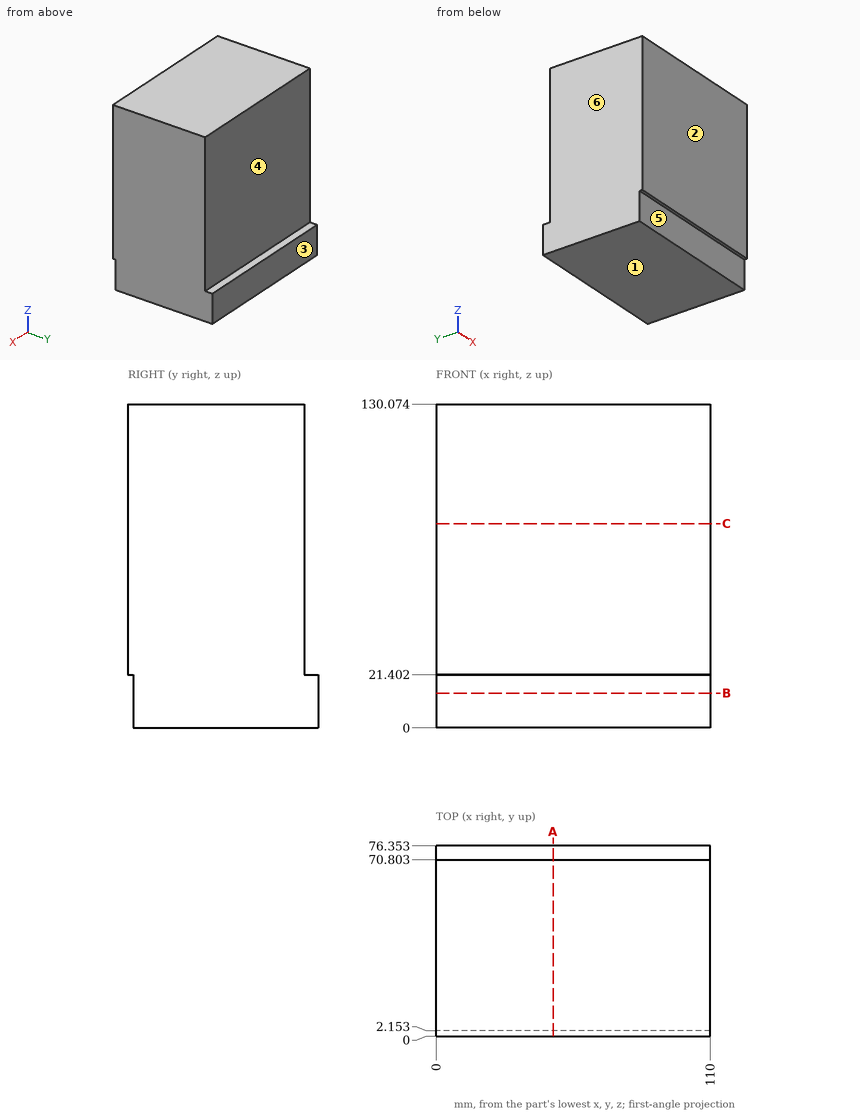
Geometry check sheet. Reference: drawing and pictorial views, mm from the part's lowest x, y, z. A direction names the side the tool comes from. Round coordinates to 2 decimals unless told otherwise and drop trailing zeros. Write each loop counter-clockwise with the first axis right and the second up, starting at its lowest first coordinate (ties: lowest second). Pieces come first, ordered by that corner, then holes.
Item 1: Section check A-A (x = 47). Record the boundary of the cut face in (y, z), plus the area to 3 significant figures.
Determined:
outline: (0, 21.4) - (2.15, 21.4) - (2.15, 0) - (76.35, 0) - (76.35, 21.4) - (70.8, 21.4) - (70.8, 130.07) - (0, 130.07) - close
area: 9,280 mm2
Item 2: Section check B-B (z = 14). Record the boundary of the cut face in (x, y).
Determined:
outline: (0, 2.15) - (110, 2.15) - (110, 76.35) - (0, 76.35) - close
Item 3: Access from +Z, -Z, +X, -X, +Y, -Y to the whole of each face (thin tool, end or side, straight path). Record for the marked faces 4, 5 and 6.
Determined:
face 4: +Z, +X, -X, +Y
face 5: -Z, +X, -X, -Y
face 6: +Z, -Z, -X, +Y, -Y
Item 4: Section check C-C (z = 82). Record the boundary of the cut face in (x, y), plus the area to 3 significant figures.
Determined:
outline: (0, 0) - (110, 0) - (110, 70.8) - (0, 70.8) - close
area: 7,790 mm2
Item 5: Go/stop test with flat-tipped pins: pin 1 Ø10.5 at (x, z) = (32, 13.5) entering from -Y; pin 2 Ø6 at (x, z) = (87, 74) entering from +Y; pin 3 Ø1.7 at (x, y) = (68, 72.5) entering from +Z. Record where each tip stops, or that it passes through.
Determined:
pin 1: stops at y = 2.15
pin 2: stops at y = 70.8
pin 3: stops at z = 21.4
Item 6: Material ranges on line 1 along Y through (x, z) = (68, 112.5); line 2 along Z through (x, y) = (92.5, 71); line 3 along Y through (x, z) = (53.5, 14), recorded low to high.
Determined:
line 1: y = 0 to 70.8
line 2: z = 0 to 21.4
line 3: y = 2.15 to 76.35
Item 7: Mould release check, pull along Y, two halves, no side actions. Record for the marked faces 1, 2 and 3: +Y half, -Y half, draft (parallel to the pull), parting line (faces both ways), or undercut.
Determined:
face 1: draft
face 2: -Y half
face 3: +Y half
